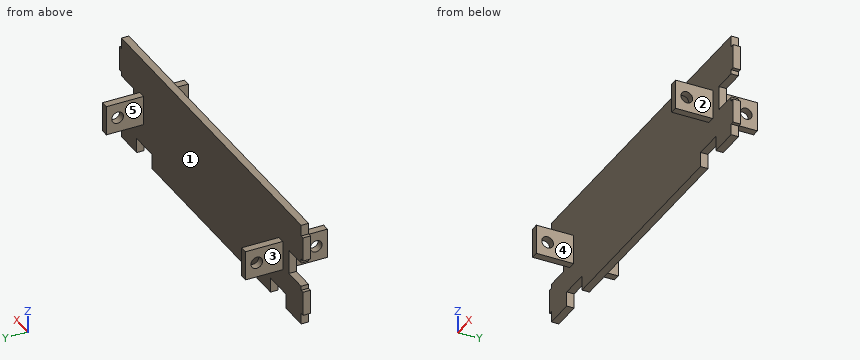
```python
from build123d import *

# Parameters (mm, degrees)
BOSS_EXTRUDE1_DEPTH     = 3.175
SKETCH2_W               = 6.35
SKETCH2_H               = 25.4
BOSS_EXTRUDE2_DEPTH     = 35.052
CUT_EXTRUDE1_DEPTH      = 277.991076082
CUT_EXTRUDE1_DEPTH_BACK = 277.991076082
SKETCH5_R               = 5.0038


with BuildPart() as part:
    # Sketch1 → Boss-Extrude1 (new, symmetric)
    with BuildSketch(Plane(origin=(0, 0, 0), x_dir=(1, 0, 0), z_dir=(0, 1, 0))):
        Polygon((149.225, -44.45), (-149.225, -44.45), (-149.225, -34.874677354), (-152.4, -34.874677354), (-152.4, -14.046677354), (-149.225, -14.046677354), (-149.225, -10.414), (-128.905, -10.414), (-128.905, 10.414), (-149.225, 10.414), (-149.225, 14.046677354), (-152.4, 14.046677354), (-152.4, 34.874677354), (-149.225, 34.874677354), (-149.225, 44.45), (-123.825, 44.45), (-123.825, 31.75), (-98.425, 31.75), (-98.425, 44.45), (98.425, 44.45), (98.425, 31.75), (123.825, 31.75), (123.825, 44.45), (149.225, 44.45), (149.225, 34.874677354), (152.4, 34.874677354), (152.4, 14.046677354), (149.225, 14.046677354), (149.225, 10.414), (128.905, 10.414), (128.905, -10.414), (149.225, -10.414), (149.225, -14.046677354), (152.4, -14.046677354), (152.4, -34.874677354), (149.225, -34.874677354), align=None)
    extrude(amount=BOSS_EXTRUDE1_DEPTH, both=True)

    # Sketch2 → Boss-Extrude2 (add, symmetric)
    with BuildSketch(Plane(origin=(0, 0, 0), x_dir=(1, 0, 0), z_dir=(0, 1, 0))):
        with Locations((115.57, 0)):
            Rectangle(SKETCH2_W, SKETCH2_H)
        with Locations((-115.57, 0)):
            Rectangle(SKETCH2_W, SKETCH2_H)
    extrude(amount=BOSS_EXTRUDE2_DEPTH, both=True)

    # Sketch5 → Cut-Extrude1 (cut, two sides: drawn at the far end of the back side and taken through both)
    with BuildSketch(Plane.ZY.offset(118.745).offset(-CUT_EXTRUDE1_DEPTH_BACK)):
        with Locations((0, 25.4)):
            Circle(SKETCH5_R)
        with Locations((0, -25.4)):
            Circle(SKETCH5_R)
    extrude(amount=CUT_EXTRUDE1_DEPTH + CUT_EXTRUDE1_DEPTH_BACK, mode=Mode.SUBTRACT)


solid = part.part
```
Verification items for the finished model (mm, model axes). Face numbers are marked on the shaded views. A direction names the side the tool comes from. Give positions to 0.01 mm unless a question says otherwise; leave off trailing zeros. Write each loop counter-clockwise with the first axis right and the second up, starting at its lowest first coordinate (ties: lowest second). Pieces come first, ordered by that corner, then holes. Notation, with made-up numbers: M -28.75,-34 L 17.25,-34 A24 cw 17.25,-17 Z; hole C 65.25,39 d7. An arc over 180 degrees is marked long. One line per question, with ' | ' between items.
1) Section check D-D on x = -11.5. Enter the section's corners in (y, z) (3 decimals).
Result:
outline: M -3.175,-44.45 L 3.175,-44.45 L 3.175,44.45 L -3.175,44.45 Z
2) Set-up check for the marked faces 4 and 5: record each of +Z, -Z, +X, -X, +Y, -Y from which the full face is reachable in a straight line by a thin tool's end or side.
Result:
face 4: +Z, -Z, -Y | face 5: +Z, -Z, +Y
3) Thickness scan on line 1 along Y through (x, z) = (-115, 0); line 2 along Z through (x, y) = (115.25, 25.4); line 3 along X through (y, z) = (32, -10.5) (3 decimals). Record the ranges inside material, lowest first. Write a range as [from, to].
Result:
line 1: y = [-35.05, -30.4], [-20.4, 20.4], [30.4, 35.05] | line 2: z = [-12.7, -5], [5, 12.7] | line 3: x = [-118.745, -112.395], [112.395, 118.745]
4) Mould release check, pull along X, two halves, no side actions. Record for the marked faces 1, 2 and 3: released by +X, released by -X, zero draft, split by the parting line, or undercut.
Result:
face 1: undercut | face 2: released by +X | face 3: released by -X
5) Section check A-A on y = 10. Enter the section's corners in (x, z) (3 decimals), plus the area to 3 significant figures.
Result:
outline: M -118.745,-12.7 L -112.395,-12.7 L -112.395,12.7 L -118.745,12.7 Z; M 112.395,-12.7 L 118.745,-12.7 L 118.745,12.7 L 112.395,12.7 Z | area: 323 mm2
6) Section check B-B on y = 25.4. Enter the section's corners in (x, z) (3 decimals).
Result:
outline: M -118.745,-12.7 L -112.395,-12.7 L -112.395,-5.004 L -118.745,-5.004 Z; M -118.745,5.004 L -112.395,5.004 L -112.395,12.7 L -118.745,12.7 Z; M 112.395,-12.7 L 118.745,-12.7 L 118.745,-5.004 L 112.395,-5.004 Z; M 112.395,5.004 L 118.745,5.004 L 118.745,12.7 L 112.395,12.7 Z
7) Section check C-C on z = 0. State how many separate pieces and enclosed holes the cut face has, plus the area to 3 significant figures.
Result:
separate pieces: 5 | enclosed holes: 0 | area: 2,190 mm2
8) Gauge pin test, flat ends, axial feed: pin 1 Ø3.5 at (x, y) = (151.5, 0.5) entering from +Z; pin 2 Ø8 at (x, y) = (17, 4) entering from +Z; pin 3 Ø4 at (y, z) = (22.5, 1) entering from -X (3 decimals); pin 4 Ø3 at (x, y) = (-29.5, 6) entering from +Z. Record the tip position at first contact, or that the pin passes through.
Result:
pin 1: stops at z = 34.87 | pin 2: stops at z = 44.45 | pin 3: stops at x = -118.745 | pin 4: passes through
